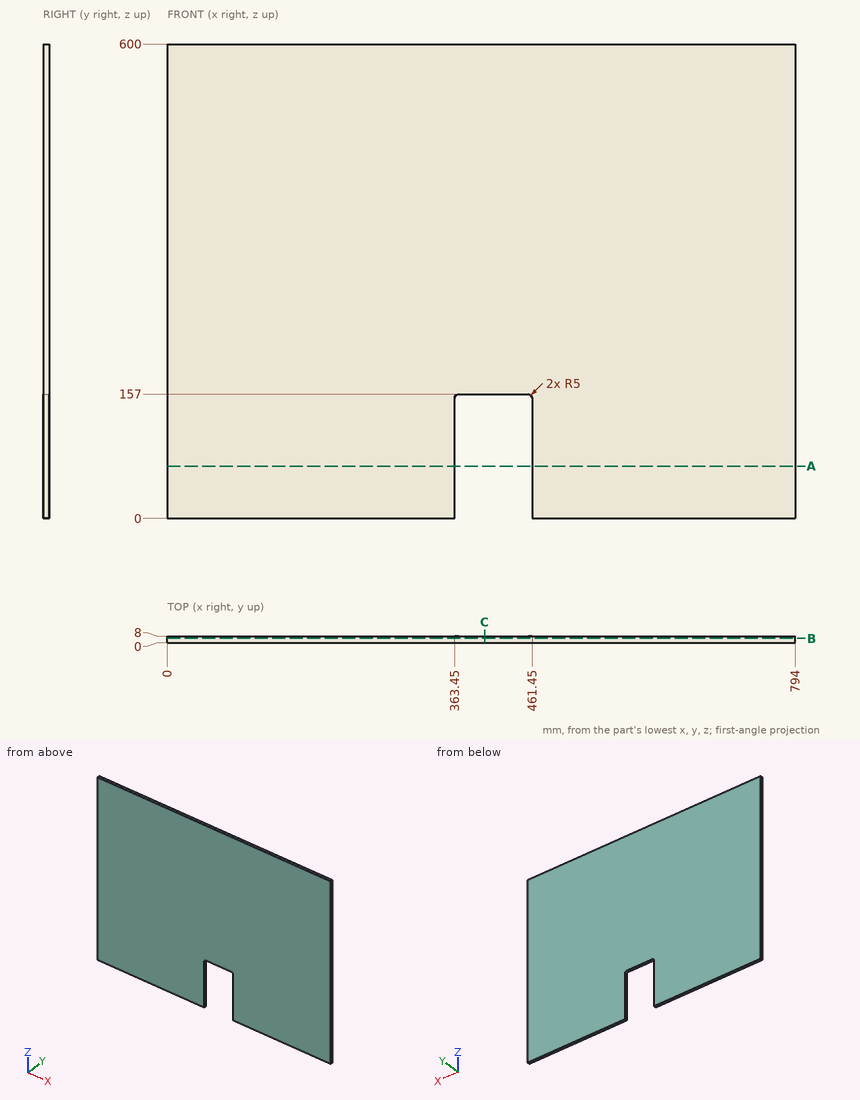
Design review of the part shown in the three views and the two pictorial views. Dimensions are in mm from the part's minimum x, y and z. Give positions to 0.01 mm unless a question says otherwise; leave off trailing zeros. Loops run counter-clockwise (first coordinate to the right, second up) from the corner with the lowest first, then second, coordinate; pieces in that order, holes last. Notation, with made-up numbers: (-22.5, -10.5) - (24.5, -10.5) arc R13 cw to (24.5, 14.5) - close; hole circle Ø7 at (-34.5, -4.75). An arc over 180 degrees is marked (long way). Answer as a JSON object with one key per item and string values.
Q1. Add section B-B on y = 5.25. State the section outline as (x, z) points, plus the area to 3 significant figures.
Worked out:
{"outline": "(0, 0) - (363.45, 0) - (363.45, 152) arc R5 cw to (368.45, 157) - (456.45, 157) arc R5 cw to (461.45, 152) - (461.45, 0) - (794, 0) - (794, 600) - (0, 600) - close", "area": "461,000 mm^2"}
Q2. Add section A-A on z = 66. State the section outline as (x, y) points.
Worked out:
{"outline": "(0, 0) - (363.45, 0) - (363.45, 8) - (0, 8) - close; (461.45, 0) - (794, 0) - (794, 8) - (461.45, 8) - close"}
Q3. Add section C-C on x = 401.5. State the section outline as (y, z) points.
Worked out:
{"outline": "(0, 157) - (8, 157) - (8, 600) - (0, 600) - close"}
Q4. To check wall thickness, follow line 1 along X through (y, z) = (7.75, 101); line 2 along X through (y, z) = (4.5, 154.5); line 3 along Z through (x, y) = (434, 2). State the ranges of each line that lie inside material, in increasing order.
Worked out:
{"line 1": "x = 0 to 363.45, 461.45 to 794", "line 2": "x = 0 to 364.12, 460.78 to 794", "line 3": "z = 157 to 600"}
